Geometry check sheet. Reference: the model listing, model coordinates, mm. Face numbers are marked on the shaded views. Coordinates: 2 decimals unless noted, no trailing zeros. Loops run counter-clockwise (first coordinate to the right, second up) from the corner with the lowest first, then second, coordinate; pieces in that order, holes last.
Autodesk Inventor part; units mm, degrees
ref_plane "Arbeitsebene1" through (0, 8, 0) normal (0, 1, 0) x (1, 0, 0)
ref_plane "YZ Plane" through (0, 0, 0) normal (1, 0, 0) x (0, 1, 0)
ref_plane "XZ Plane" through (0, 0, 0) normal (0, 1, 0) x (-1, 0, 0)
sketch "Skizze1" plane through (0, 0, 0) normal (0, 1, 0) x (-1, 0, 0)
  line L0 (0, 0) -> (-90, 0)
  line L1 (-90, 0) -> (-90, -158)
  line L2 (-90, -158) -> (0, -158)
  line L3 (0, -158) -> (0, 0)
  line L4 (18, 18) -> (-168, 18)
  line L5 (-168, 18) -> (-168, -218)
  line L6 (-168, -218) -> (18, -218)
  line L7 (18, -218) -> (18, 18)
  circle A0 centre (8, 5.5) radius 2.5
  circle A1 centre (10, -207) radius 2.5
  circle A2 centre (-158, -208.5) radius 2.5
  circle A3 centre (-160, 4.5) radius 2.5
  dimension "d0" = 90
  dimension "d1" = 158
  dimension "d2" = 78
  dimension "d3" = 18
  dimension "d4" = 18
  dimension "d5" = 60
  dimension "r" = 5
  dimension "d7" = 5
  dimension "d8" = 5
  dimension "d9" = 5
  dimension "d10" = 8
  dimension "d11" = 5.5
  dimension "d12" = 4.5
  dimension "d13" = 70
  dimension "d14" = 68
  dimension "d15" = 50.5
  dimension "d16" = 49
  dimension "d17" = 10
extrude "Extrusion1" add sketch "Skizze1" along normal blind 4
fillet "Rundung1" radius 3 4 edges at (-18, 2, -218) (-18, 2, 18) (168, 2, 18) (168, 2, -218)
ref_plane "Arbeitsebene1" through (0, 8, 0) normal (0, 1, 0) x (1, 0, 0)
sketch "Skizze3" plane through (0, 4, 0) normal (0, 1, 0) x (1, 0, 0)
  line L0 (112.9385, 54.4149) -> (112.9385, 81.7299)
  line L1 (112.9385, 81.7299) -> (146.9954, 81.7299) construction
  line L2 (146.9954, 81.7299) -> (146.9954, 54.4149) construction
  line L3 (146.9954, 54.4149) -> (112.9385, 54.4149) construction
  line L4 (112.9385, 54.4149) -> (146.9954, 54.4149)
  line L5 (146.9954, 54.4149) -> (146.9954, 81.7299)
  line L6 (146.9954, 81.7299) -> (112.9385, 81.7299)
  line L7 (112.9385, 81.7299) -> (112.9385, 54.4149)
  point P0 (0, 0)
extrude "Extrusion3" cut sketch "Skizze3" against normal blind 2
equation "\"d7\" = r"
equation "\"d8\" = r"
equation "\"d9\" = r"
equation "\"d50\" = a"
equation "\"d51\" = a"
equation "\"d52\" = a"
properties part number "frontpanel"
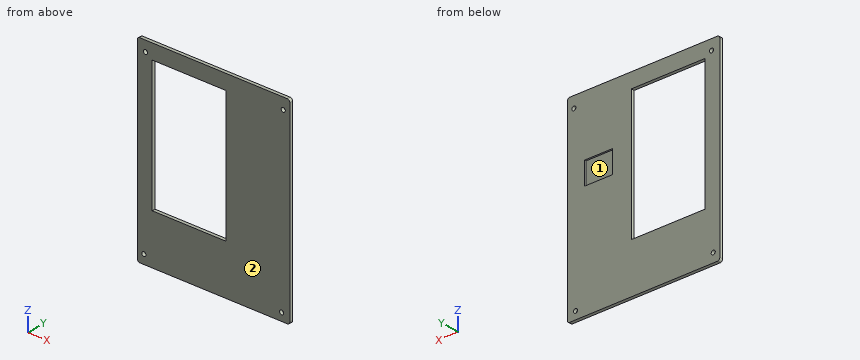
(1) Sectioned sample at D-D on z = -61. Record the cut outline in (x, y), and give its area (3 significant figures).
Findings:
outline: (-18, 0) - (0, 0) - (0, 4) - (-18, 4) - close; (90, 0) - (168, 0) - (168, 4) - (147, 4) - (147, 2) - (112.94, 2) - (112.94, 4) - (90, 4) - close
area: 316 mm2
(2) Scan lines: L1, parallel to Z at x = -10, y = 2.1; L2, parallel to X at y = 3.85, z = -152.5; L3, parallel to Z at x = 145, y = 2.45. Record each from-to range of solid material in increasing order.
Findings:
L1: z = -218 to -209.5, -204.5 to 4, 7 to 18
L2: x = -18 to 0, 90 to 168
L3: z = -218 to -81.73, -54.41 to 18
(3) Gauge pin test, flat ends, axial feed: pin 1 Ø8 at (x, z) = (137, -69) entering from +Y; pin 2 Ø3 at (x, z) = (-10, -207) entering from +Y. Record the tip position at first contact, or that the pin passes through.
Findings:
pin 1: stops at y = 2
pin 2: passes through
(4) Sectioned sample at B-B on y = 3.3. Record the cut outline in (x, z).
Findings:
outline: (-18, -215) arc R3 ccw to (-15, -218) - (165, -218) arc R3 ccw to (168, -215) - (168, 15) arc R3 ccw to (165, 18) - (-15, 18) arc R3 ccw to (-18, 15) - close; hole circle Ø5 at (-10, -207); hole circle Ø5 at (-8, 5.5); hole (0, -158) - (90, -158) - (90, 0) - (0, 0) - close; hole (112.94, -81.73) - (147, -81.73) - (147, -54.41) - (112.94, -54.41) - close; hole circle Ø5 at (158, -208.5); hole circle Ø5 at (160, 4.5)
(5) Sectioned sample at C-C on x = 59. Record the cut outline in (y, z).
Findings:
outline: (0, -218) - (4, -218) - (4, -158) - (0, -158) - close; (0, 0) - (4, 0) - (4, 18) - (0, 18) - close
(6) Sectioned sample at A-A on z = -147.5. Record the cut outline in (x, y), and give its area (3 significant figures).
Findings:
outline: (-18, 0) - (0, 0) - (0, 4) - (-18, 4) - close; (90, 0) - (168, 0) - (168, 4) - (90, 4) - close
area: 384 mm2
(7) Draft check along X on the marked faces 1 and 2. Enter one of: +X half, -X half, draft (parallel to the pull), parting line (faces both ways), or undercut.
Findings:
face 1: undercut
face 2: draft
